For this review, use the dimensioned drawing (mm, ordinates from the lowest corner) and the shaded views. A direction names the side the tool comes from. Coordinates: 2 decimals unless noted, no trailing zeros. Write each loop counter-clockwise with the first axis right and the second up, starting at its lowest first coordinate (ties: lowest second). Pieces come first, ordered by that corner, then holes. Notation, with made-up numbers: (83.25, 86) -> (101.25, 86) arc R22 cw to (101.25, 123) -> close; hole circle Ø7 at (22, 54.5). An arc over 180 degrees is marked (long way). Return JSON: item names as keys, results as strings. Group by question number.
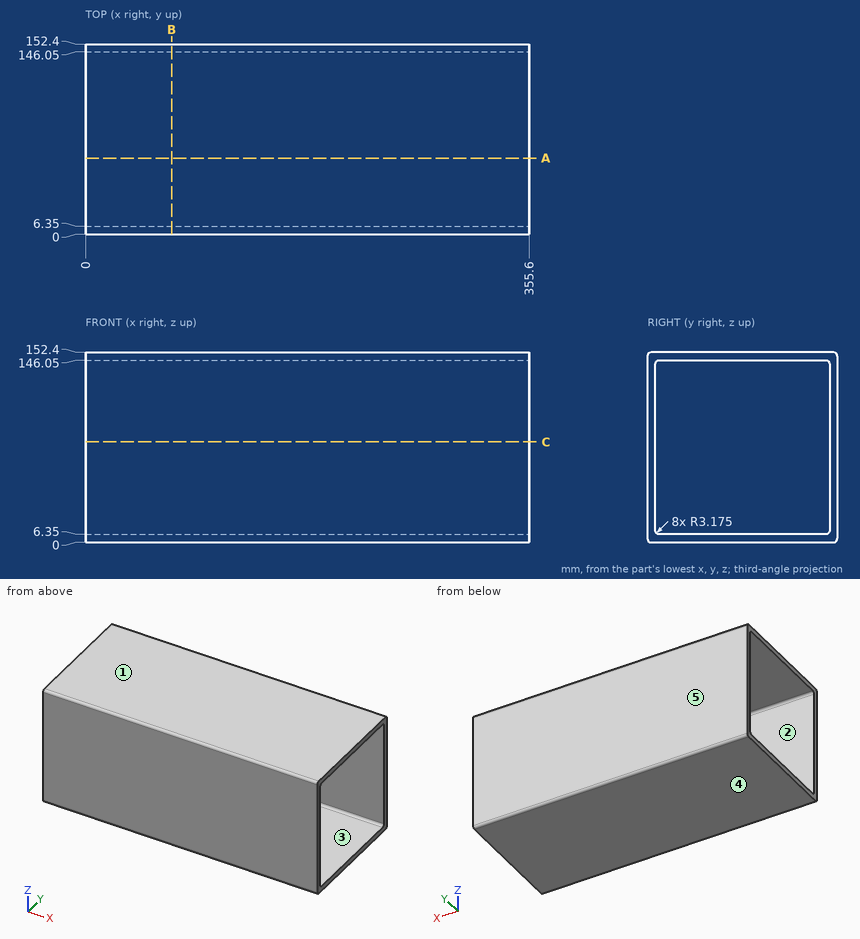
Q1. For the marked faces 1 and 2, list the 3-axis set-ups (+Z, -Z, +X, -X, +Y, -Y) from which the entire face can be reached by the end or side of a thin tool; tool diameter is ignored.
Q2. The part is to be moulded in two halves that separate along Y. For the marked faces 3, 4 and 5, say which applies: +Y half, -Y half, draft (parallel to the pull), parting line (faces both ways), or undercut.
Q3. We need section B-B on x = 69. Write out the cut boundary in (y, z) (3 decimals), plus the area to 3 significant figures.
Q4. Wall thickness on L1, parallel to Z at x = 150, y = 66; L2, parallel to Y at x = 80, z = 7.5: over which ranges is each line inside the solid? List them lowest first.
Q5. We need section A-A on y = 61. Write out the cut boundary in (x, z), plus the area to 3 significant figures.
Findings below:
{
 "1": {"face 1": "+Z, +X, -X, +Y, -Y", "face 2": "+X, -X"},
 "2": {"face 3": "undercut", "face 4": "draft", "face 5": "+Y half"},
 "3": {"outline": "(0, 3.175) arc R3.175 ccw to (3.175, 0) -> (149.225, 0) arc R3.175 ccw to (152.4, 3.175) -> (152.4, 149.225) arc R3.175 ccw to (149.225, 152.4) -> (3.175, 152.4) arc R3.175 ccw to (0, 149.225) -> close; hole (6.35, 9.525) arc R3.175 ccw to (9.525, 6.35) -> (142.875, 6.35) arc R3.175 ccw to (146.05, 9.525) -> (146.05, 142.875) arc R3.175 ccw to (142.875, 146.05) -> (9.525, 146.05) arc R3.175 ccw to (6.35, 142.875) -> close", "area": "3,710 mm^2"},
 "4": {"L1": "z = 0 to 6.35, 146.05 to 152.4", "L2": "y = 0 to 7.08, 145.32 to 152.4"},
 "5": {"outline": "(0, 0) -> (355.6, 0) -> (355.6, 6.35) -> (0, 6.35) -> close; (0, 146.05) -> (355.6, 146.05) -> (355.6, 152.4) -> (0, 152.4) -> close", "area": "4,520 mm^2"}
}
